The model under review builds one solid part; all positions refer to its coordinate system, in mm. Coordinates: 2 decimals unless noted, no trailing zeros. Order: outer loops, then holes, each group sorted by start corner. A loop starts at its lowest first (then second) coordinate and runs counter-clockwise, first axis right, second up. Notation, with made-up numbers: (42.25, -3) -> (56.25, -3) arc R22 cw to (56.25, 10) -> close; hole circle Ø3 at (-10.75, 27.25). An arc over 180 degrees is marked (long way). Use one line per item in the form item = value.
from build123d import *

# Parameters (mm, degrees)
F0_R     = 0.7
F1_DEPTH = 55
F3_DEPTH = 70


# Not quite as in the source:
# - a feature of the source that left no trace in its solid (it failed there, or was rolled back) is left out


with BuildPart() as f1:
    # F0 (on Front) → F1 (new body)
    with BuildSketch(Plane.XZ):
        Circle(F0_R)
    extrude(amount=F1_DEPTH)

    # F2 (on Front) → F3 (join)
    with BuildSketch(Plane.XZ):
        with BuildLine():
            Line((1.5, -2.5), (1.5, 2.5))
            Line((1.5, 2.5), (0, 2.5))
            ThreePointArc((0, 2.5), (-0.4472135955, 2.394427191), (-0.8, 2.1))
            ThreePointArc((-0.8, 2.1), (-1.5, 0), (-0.8, -2.1))
            ThreePointArc((-0.8, -2.1), (-0.4472135955, -2.394427191), (0, -2.5))
            Line((0, -2.5), (1.5, -2.5))
        make_face()
    extrude(amount=-F3_DEPTH)


solid = f1.part
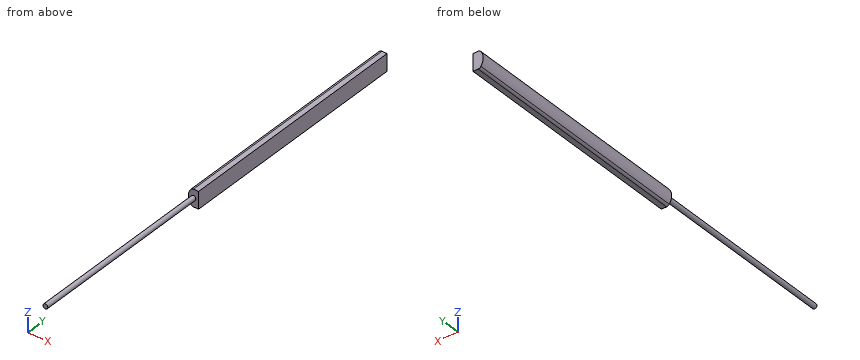
Item 1: Clearance check with a flat-ended pin moving along its axis: pin 1 (1 mm diameter, centred on x = -1, y = 28.5, fed in from +Z). State where the tip first meets the part, or that it passes through.
Results found:
pin_1 = 2.37
Item 2: We need section A-A (y = -39). Write out the cut boundary in (x, z), plus the area to 3 significant figures.
Results found:
outline = circle Ø1.4 at (0, 0)
area = 1.54 mm²
Item 3: To check wall thickness, follow L1, parallel to X at y = 64, z = -0.2; L2, parallel to Y at x = -0.35, z = 2.1; L3, parallel to Z at x = -0.05, y = 27. State the ranges of each line that lie inside material, in increasing order. Write a range as from..to.
Results found:
L1 = -1.49..1.5
L2 = 0..70
L3 = -2.5..2.5
